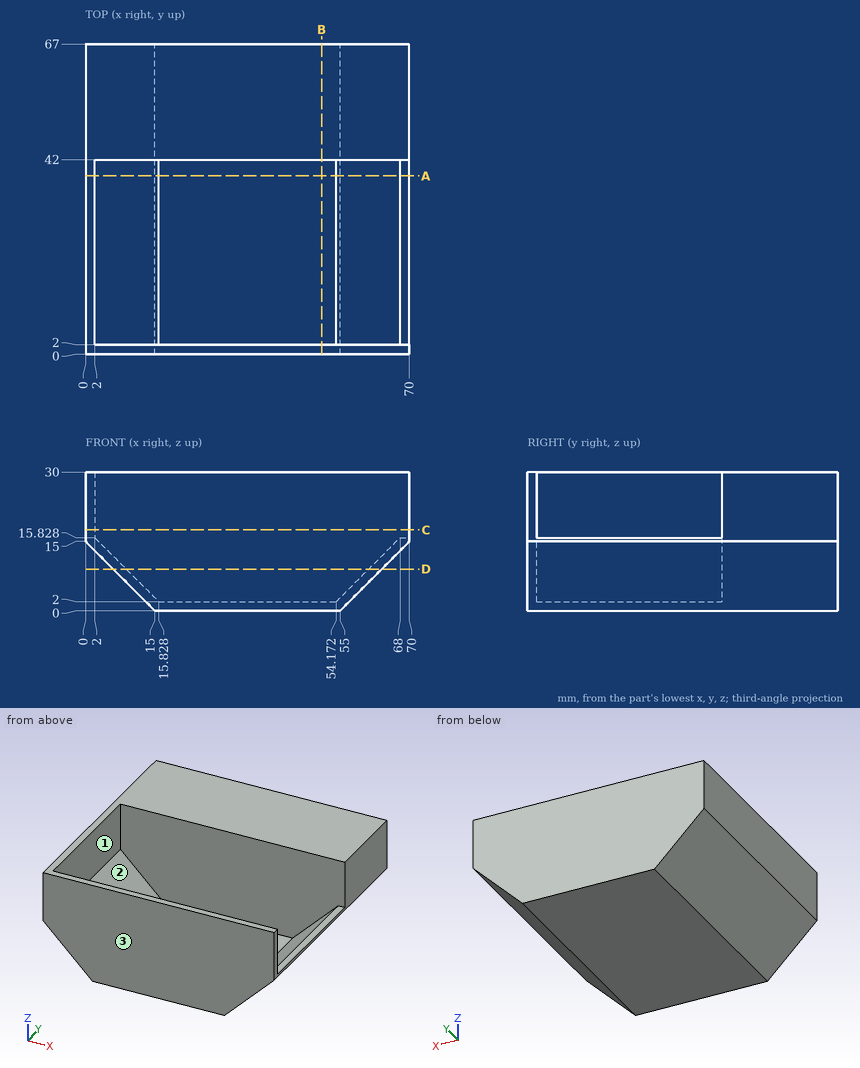
The drawing under review shows one solid part. Ordinate dimensions are in mm from its lowest x, y, z. A direction names the side the tool comes from. Coordinates: 2 decimals unless noted, no trailing zeros. Loops run counter-clockwise (first coordinate to the right, second up) from the corner with the lowest first, then second, coordinate; pieces in that order, holes last.
Item 1: Wall thickness on L1, parallel to Y at x = 28, z = 9; L2, parallel to Z at x = 26, y = 11.5; L3, parallel to X at y = 5, z = 14: over which ranges is each line inside the solid? List them lowest first.
Completed:
L1: y = 0 to 2, 42 to 67
L2: z = 0 to 2
L3: x = 1 to 3.83, 66.17 to 69
Item 2: Clearance check with flat-ended pins moving along their axes: pin 1 (1 mm diameter, centred on x = 7.5, z = 6, fed in from +Y); pin 2 (0.6 mm diameter, centred on x = 69, y = 27.5, fed in from +Z); pin 3 (11.5 mm diameter, centred on x = 33.5, y = 12, fed in from +Z); pin 4 (3 mm diameter, centred on y = 58.5, z = 12, fed in from -X). State where each tip first meets the part, or that it passes through.
Completed:
pin 1: passes through
pin 2: stops at z = 15.83
pin 3: stops at z = 2
pin 4: stops at x = 1.5
Item 3: Add section B-B (x = 51). Write out the cut boundary in (y, z), and give its area (3 significant figures).
Completed:
outline: (0, 0) - (67, 0) - (67, 30) - (42, 30) - (42, 2) - (2, 2) - (2, 30) - (0, 30) - close
area: 890 mm2
Item 4: For the marked faces 1, 2 and 3, list the 3-axis set-ups (+Z, -Z, +X, -X, +Y, -Y) from which the entire face can be reached by the end or side of a thin tool; tool diameter is ignored.
Completed:
face 1: +Z, +X
face 2: +Z
face 3: +Z, -Z, +X, -X, -Y
Item 5: Add section D-D (z = 9). Write out the cut boundary in (x, y), and give its area (3 significant figures).
Completed:
outline: (6, 0) - (64, 0) - (64, 67) - (6, 67) - close; hole (8.83, 2) - (61.17, 2) - (61.17, 42) - (8.83, 42) - close
area: 1,790 mm2
Item 6: Add section C-C (z = 17.5). Write out the cut boundary in (x, y), and give its area (3 significant figures).
Completed:
outline: (0, 0) - (70, 0) - (70, 2) - (2, 2) - (2, 42) - (70, 42) - (70, 67) - (0, 67) - close
area: 1,970 mm2
Item 7: Add section A-A (y = 38.5). Write out the cut boundary in (x, z), and give its area (3 significant figures).
Completed:
outline: (0, 15) - (15, 0) - (55, 0) - (70, 15) - (70, 15.83) - (68, 15.83) - (54.17, 2) - (15.83, 2) - (2, 15.83) - (2, 30) - (0, 30) - close
area: 190 mm2
